Geometry: see drawing. Coordinates: mm, zero at the bounding-box minimum. A direction names the side the tool comes from. Give positions to 0.01 mm unless a question says otherwise; leave off trailing zeros. Write each loop counter-clockwise with the first axis right and the second up, starting at its lowest first coordinate (ties: lowest second). Pieces come first, ordered by that corner, then holes. Notation, with made-up numbers: (-2, -2.5) - (11, -2.5) arc R35 ccw to (11, 31.5) - close; hole circle Ø11 at (85, 78.5). An arc over 180 degrees is marked (long way). Use CSV: the item, a comma, the result in double quotes. Start each with the question number.
(1) Section A-A on z = 35. Output: boundary loops of the cut face in (x, y), and give its area (3 significant figures).
(2) Reachability of the marked faces 5 and 6 from +Z, -Z, +X, -X, +Y, -Y: full face, straight path, thin tool, end or side. Return the list, or none.
(3) Section C-C on y = 20. Output: boundary loops of the cut face in (x, z).
(4) Section B-B on x = 3. Output: boundary loops of the cut face in (y, z), and give its area (4 significant figures).
(5) First-contact query: pin 1 Ø1.5 at (x, z) = (9.5, 18) entering from +Y; pin 2 Ø10 at (x, y) = (9, 20.5) entering from +Z. Flat tips, straight axial feed; report the tip coordinate or a pass-through.
(6) Section D-D on x = 10. Output: boundary loops of the cut face in (y, z), and give its area (3 significant figures).
(7) Line query: probe 1 along X at (y, z) = (20, 2.3); probe 2 along Z at (x, y) = (17, 2.85); probe 3 along Y at (x, z) = (10, 4.05). Output: solid intervals per line, ascending. Write a range as [from, to].
(8) Draft query along Y for the marked faces 1, 2, 3 and 4. Return one class per face: released by +Y, released by -Y, zero draft, split by the parting line, or undercut.
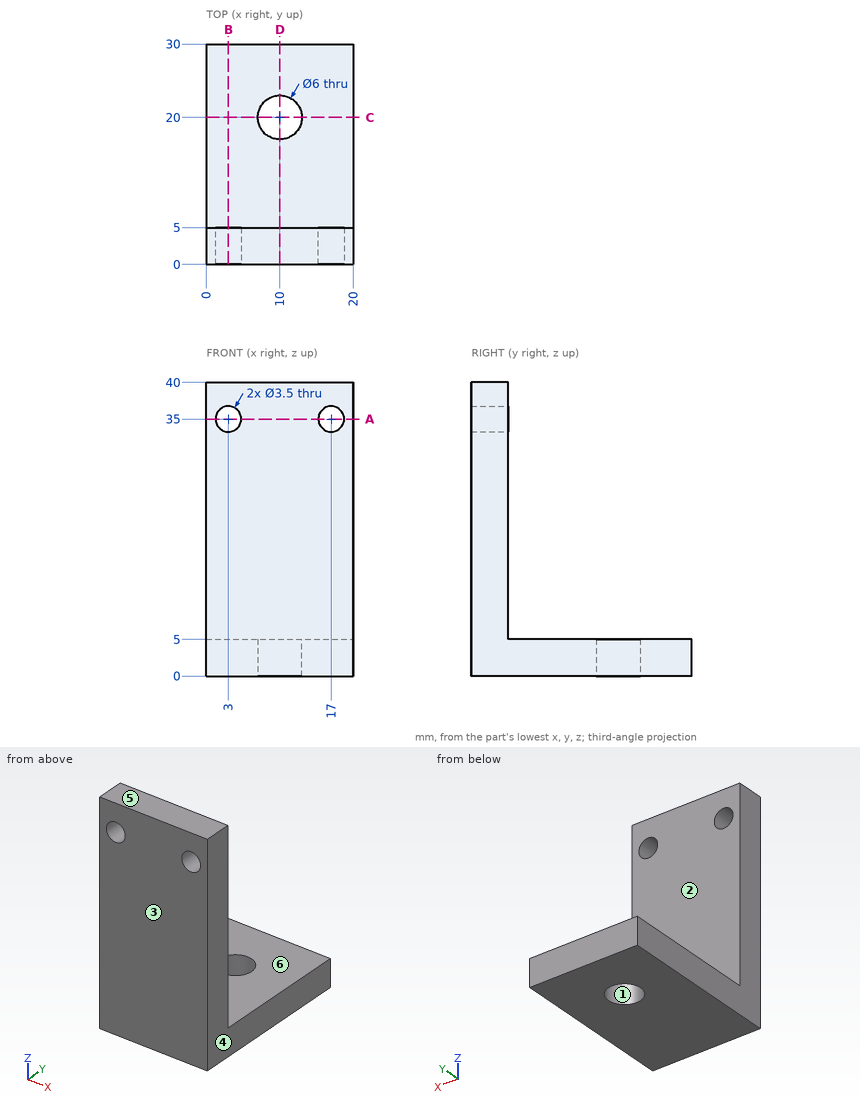
Check values:
1,outline,"(0, 0) - (1.25, 0) - (1.25, 5) - (0, 5) - close; (4.75, 0) - (15.25, 0) - (15.25, 5) - (4.75, 5) - close; (18.75, 0) - (20, 0) - (20, 5) - (18.75, 5) - close"
1,area,"65.0 mm²"
2,face 5,"+Z, +X, -X, +Y, -Y"
2,face 6,"+Z, +X, -X, +Y"
3,outline,"(0, 0) - (7, 0) - (7, 5) - (0, 5) - close; (13, 0) - (20, 0) - (20, 5) - (13, 5) - close"
4,outline,"(0, 0) - (30, 0) - (30, 5) - (5, 5) - (5, 33.25) - (0, 33.25) - close; (0, 36.75) - (5, 36.75) - (5, 40) - (0, 40) - close"
4,area,"307.5 mm²"
5,pin 1,"stops at y = 5"
5,pin 2,"stops at z = 5"
6,outline,"(0, 0) - (17, 0) - (17, 5) - (5, 5) - (5, 40) - (0, 40) - close; (23, 0) - (30, 0) - (30, 5) - (23, 5) - close"
6,area,"295 mm²"
7,probe 1,"x = [0, 7], [13, 20]"
7,probe 2,"z = [0, 33.25], [36.75, 40]"
7,probe 3,"y = [0, 17], [23, 30]"
8,face 1,"undercut"
8,face 2,"released by +Y"
8,face 3,"released by -Y"
8,face 4,"zero draft"
